For this review, take the finished solid that the model builds, in its own axes (mm). Give positions to 0.01 mm unless a question says otherwise; leave off trailing zeros. Order: outer loops, then holes, each group sorted by start corner. A loop starts at its lowest first (then second) coordinate and runs counter-clockwise, first axis right, second up.
Item 1: Consider section B-B (z = 5). Give the boundary of the cut face in (x, y), plus the area to 3 significant figures.
Item 2: Consider section A-A (y = 0.51). Give the boundary of the cut face in (x, z).
Item 3: For probe 1 along X at (y, z) = (0.51, 6); probe 2 along Z at (x, y) = (-29.35, -3.25); probe 3 along X at (y, z) = (-0.5, 8.25), list the stretches that pass through material, from the lowest coordinate up.
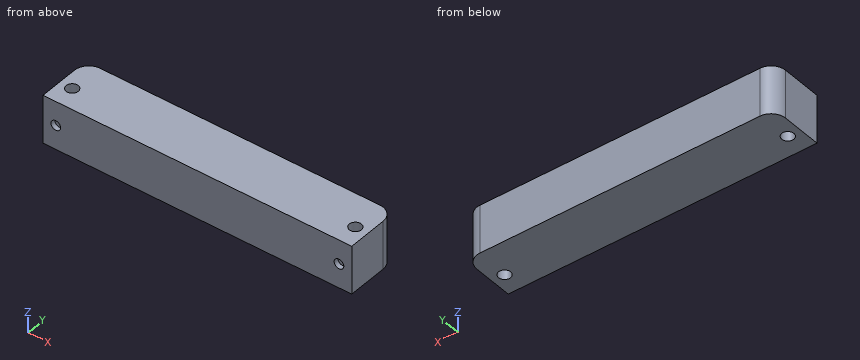
```python
from build123d import *

# Parameters (mm, degrees)
SKETCH_W        = 64
SKETCH_H        = 11.3
PAD_DEPTH       = 10
SKETCH004_R     = 1
POCKET_DEPTH    = 1
SKETCH006_R     = 1.25
POCKET002_DEPTH = 10.001
FILLET001_R     = 3


with BuildPart() as part:
    # Sketch → Pad (new body)
    with BuildSketch(Plane.XY):
        with Locations((0, 5.65)):
            Rectangle(SKETCH_W, SKETCH_H)
    extrude(amount=PAD_DEPTH)

    # Sketch004 (on Face3 of Pad) → Pocket (cut)
    with BuildSketch(Plane.XZ):
        with Locations((29.35, 5)):
            Circle(SKETCH004_R)
        with Locations((-29.35, 5)):
            Circle(SKETCH004_R)
    extrude(amount=-POCKET_DEPTH, mode=Mode.SUBTRACT)

    # Sketch006 (on Face4 of Pocket) → Pocket002 (cut, through all)
    with BuildSketch(Plane(origin=(0, 0, 0), x_dir=(1, 0, 0), z_dir=(0, 0, -1))):
        with Locations((29.35, -4.35)):
            Circle(SKETCH006_R)
        with Locations((-29.35, -4.35)):
            Circle(SKETCH006_R)
    extrude(amount=-POCKET002_DEPTH, mode=Mode.SUBTRACT)

    # Fillet001
    fillet001_edges = [part.edges().sort_by_distance(p)[0] for p in [
        (-32, 11.3, 5),
        (32, 11.3, 5),
    ]]
    fillet(fillet001_edges, radius=FILLET001_R)


with BuildPart() as part_1:
    # Body placement: moved
    add(part.part.moved(Location((0, -3.84, 0))))


solid = part_1.part
```
Resolved:
1. outline: (-32, -3.84) - (-30.35, -3.84) - (-30.35, -2.84) - (-28.35, -2.84) - (-28.35, -3.84) - (28.35, -3.84) - (28.35, -2.84) - (30.35, -2.84) - (30.35, -3.84) - (32, -3.84) - (32, 4.46) arc R3 ccw to (29, 7.46) - (-29, 7.46) arc R3 ccw to (-32, 4.46) - close; hole circle Ø2.5 at (-29.35, 0.51); hole circle Ø2.5 at (29.35, 0.51)
1. area: 706 mm2
2. outline: (-32, 0) - (-30.6, 0) - (-30.6, 10) - (-32, 10) - close; (-28.1, 0) - (28.1, 0) - (28.1, 10) - (-28.1, 10) - close; (30.6, 0) - (32, 0) - (32, 10) - (30.6, 10) - close
3. probe 1: x = -32 to -30.6, -28.1 to 28.1, 30.6 to 32
3. probe 2: z = 0 to 4, 6 to 10
3. probe 3: x = -32 to -30.09, -28.61 to 28.61, 30.09 to 32
